Geometry check sheet. Reference: the model listing, model coordinates, mm. A direction names the side the tool comes from. Give positions to 0.01 mm unless a question says otherwise; leave off trailing zeros. Write each loop counter-clockwise with the first axis right and the second up, starting at its lowest first coordinate (ties: lowest second). Pieces come first, ordered by that corner, then holes.
(1) Cross-section at A-A (y = 13). Record the boundary of the cut face in (x, z).
(2) Mould release check, pull along X, two halves, no side actions. Record for faces 1 (the flat face through (-4, 36.037, 2)), 2 (the flat face through (-39.937, 18, 2)), 3 (the flat face through (11, 5.537, 1)), 4 (the flat face through (-3, 31.843, 1)): +X half, -X half, draft (parallel to the pull), parting line (faces both ways), or undercut.
(3) Thickness scan on line 1 along X through (y, z) = (13.5, 0.75); line 2 along Y through (x, z) = (0, 3.35); line 3 along X through (y, z) = (32.5, 0.8). Record the ranges inside material, lowest first.
(4) Cross-section at B-B (x = -14). Record the boundary of the cut face in (y, z).
(5) Depth check by flat-ended pin: P1, Ø3.5, axis at x = -17.22, y = 30.78, coming from the -Z side; P2, Ø12, axis at x = -14.5, y = 17.5, coming from the +Z side; P3, Ø0.8, axis at x = -26, z = 4, coming from the -Y side; P4, Ø0.5, axis at y = 24.5, z = 4, coming from the -X side. Enter the tip coordinate at first touch or a pass-through.
(6) Cross-section at D-D (x = 25). Record the boundary of the cut face in (y, z), and give its area (3 significant figures).
(7) Cross-section at C-C (z = 2.4). Record the boundary of the cut face in (x, y).
(8) Tool access check on faces 5 (the flat face through (-28, 23, 4.5)), 6 (the flat face through (-19.817, 17, 2)), 7 (the flat face through (-19.582, 17, 1)), 8 (the flat face through (-37, 1.037, 2)). Record the directions out of +Z, -Z, +X, -X, +Y, -Y that give a thin tool (end or side, any length) a straight path to the whole face; none if there is none.
```python
from build123d import *

# Parameters (mm, degrees)
SKETCH3_R           = 1.4
SKETCH3_R_2         = 1
BOSS_EXTRUDE1_DEPTH = 3.5
SKETCH9_W           = 33.2
SKETCH9_H           = 33.2
CUT_EXTRUDE1_DEPTH  = 2.2
SKETCH10_W          = 20
SKETCH10_H          = 2.5
CUT_EXTRUDE2_DEPTH  = 1.75
SKETCH11_R          = 1
BOSS_EXTRUDE2_DEPTH = 1
SKETCH14_R          = 3.1
CUT_EXTRUDE3_DEPTH  = 1
SKETCH15_W          = 6.5
SKETCH15_H          = 2
CUT_EXTRUDE4_DEPTH  = 54.906325173


with BuildPart() as part:
    # Sketch3 → Boss-Extrude1 (new body)
    with BuildSketch(Plane.XY):
        Polygon((-39.936821352, -0.962627815), (-39.936821352, 36.037372185), (33.503178648, 36.037372185), (33.503178648, -0.962627815), (7.298178648, -0.962627815), (-14.831821352, -0.962627815), align=None)
        with Locations((-17.216821352, 30.777902568)):
            Circle(SKETCH3_R, mode=Mode.SUBTRACT)
        with Locations((-36.936821352, 32.642902568)):
            Circle(SKETCH3_R_2, mode=Mode.SUBTRACT)
        with Locations((-23.426821352, 32.642902568)):
            Circle(SKETCH3_R_2, mode=Mode.SUBTRACT)
        with Locations((16.993178648, 32.642902568)):
            Circle(SKETCH3_R_2, mode=Mode.SUBTRACT)
        with Locations((30.503178648, 32.642902568)):
            Circle(SKETCH3_R_2, mode=Mode.SUBTRACT)
        with Locations((-17.216821352, 2.777902568)):
            Circle(SKETCH3_R, mode=Mode.SUBTRACT)
        with Locations((10.783178648, 30.777902568)):
            Circle(SKETCH3_R, mode=Mode.SUBTRACT)
        with Locations((10.783178648, 2.777902568)):
            Circle(SKETCH3_R, mode=Mode.SUBTRACT)
        Polygon((-14.981821352, 0.537372185), (-14.981821352, 5.537372185), (-19.581821352, 5.537372185), (-19.581821352, 27.842902568), (-14.981821352, 27.842902568), (-14.981821352, 29.342902568), (8.548178648, 29.342902568), (8.548178648, 27.842902568), (13.148178648, 27.842902568), (13.148178648, 5.537372185), (8.548178648, 5.537372185), (8.548178648, 0.537372185), align=None, mode=Mode.SUBTRACT)
    extrude(amount=BOSS_EXTRUDE1_DEPTH)

    # Sketch9 → Cut-Extrude1 (cut)
    with BuildSketch(Plane(origin=(0, 0, 3.5), x_dir=(-1, 0, 0), z_dir=(0, 0, -1))):
        with Locations((3.216821352, 16.777902568)):
            Rectangle(SKETCH9_W, SKETCH9_H)
    extrude(amount=CUT_EXTRUDE1_DEPTH, mode=Mode.SUBTRACT)

    # Sketch10 → Cut-Extrude2 (cut)
    with BuildSketch(Plane(origin=(0, 0, 0), x_dir=(-1, 0, 0), z_dir=(0, 0, -1))):
        with Locations((3.216821352, 30.592902568)):
            Rectangle(SKETCH10_W, SKETCH10_H)
    extrude(amount=-CUT_EXTRUDE2_DEPTH, mode=Mode.SUBTRACT)

    # Sketch11 → Boss-Extrude2 (add)
    with BuildSketch(Plane.XY.offset(3.5)):
        with BuildLine():
            Line((-34.636821352, 30.942902568), (-34.636821352, 10.942902568))
            Line((-34.636821352, 10.942902568), (-22.636821352, 10.942902568))
            Line((-22.636821352, 10.942902568), (-22.636821352, 30.942902568))
            Line((-22.636821352, 30.942902568), (-21.751928528, 30.942902568))
            ThreePointArc((-21.751928528, 30.942902568), (-21.800520269, 31.226847518), (-21.826821352, 31.513717078))
            Line((-21.826821352, 31.513717078), (-21.826821352, 34.342902568))
            Line((-21.826821352, 34.342902568), (-34.636821352, 34.342902568))
            Line((-34.636821352, 34.342902568), (-34.636821352, 30.942902568))
        make_face()
        with Locations((-23.426821352, 32.642902568)):
            Circle(SKETCH11_R, mode=Mode.SUBTRACT)
    boss_extrude2 = extrude(amount=BOSS_EXTRUDE2_DEPTH)

    # Mirror1: Boss-Extrude2 across plane
    add(boss_extrude2.mirror(Plane.ZY.offset(3.216821352)))

    # Sketch14 → Cut-Extrude3 (cut)
    with BuildSketch(Plane.XY.offset(4.5)):
        with Locations((17.142214959, 27.392343087)):
            Circle(SKETCH14_R)
    extrude(amount=-CUT_EXTRUDE3_DEPTH, mode=Mode.SUBTRACT)

    # Sketch15 → Cut-Extrude4 (cut, through all)
    with BuildSketch(Plane.XY.offset(3.5)):
        with Locations((-36.686821352, 0.037372185)):
            Rectangle(SKETCH15_W, SKETCH15_H)
        with Locations((30.253178648, 0.037372185)):
            Rectangle(SKETCH15_W, SKETCH15_H)
    extrude(amount=-CUT_EXTRUDE4_DEPTH, mode=Mode.SUBTRACT)


solid = part.part
```
Reply:
1. outline: (-39.94, 0) - (-19.58, 0) - (-19.58, 1.3) - (-19.82, 1.3) - (-19.82, 3.5) - (-22.64, 3.5) - (-22.64, 4.5) - (-34.64, 4.5) - (-34.64, 3.5) - (-39.94, 3.5) - close; (13.15, 0) - (33.5, 0) - (33.5, 3.5) - (28.2, 3.5) - (28.2, 4.5) - (16.2, 4.5) - (16.2, 3.5) - (13.38, 3.5) - (13.38, 1.3) - (13.15, 1.3) - close
2. face 1: draft
2. face 2: -X half
2. face 3: undercut
2. face 4: undercut
3. line 1: x = -39.94 to -19.58, 13.15 to 33.5
3. line 2: y = -0.96 to 0.18, 33.38 to 36.04
3. line 3: x = -39.94 to -37.93, -35.95 to -24.42, -22.44 to 16, 17.98 to 29.51, 31.49 to 33.5
4. outline: (-0.96, 0) - (0.54, 0) - (0.54, 1.3) - (0.18, 1.3) - (0.18, 3.5) - (-0.96, 3.5) - close; (29.34, 0) - (36.04, 0) - (36.04, 3.5) - (33.38, 3.5) - (33.38, 1.3) - (29.34, 1.3) - close
5. P1: stops at z = 0
5. P2: stops at z = 3.5
5. P3: stops at y = 10.94
5. P4: stops at x = -34.64
6. outline: (-0.96, 0) - (36.04, 0) - (36.04, 3.5) - (34.34, 3.5) - (34.34, 4.5) - (10.94, 4.5) - (10.94, 3.5) - (-0.96, 3.5) - close
6. area: 153 mm2
7. outline: (-39.94, 1.04) - (-33.44, 1.04) - (-33.44, -0.96) - (27, -0.96) - (27, 1.04) - (33.5, 1.04) - (33.5, 36.04) - (-39.94, 36.04) - close; hole circle Ø2 at (-36.94, 32.64); hole circle Ø2 at (-23.43, 32.64); hole (-19.82, 0.18) - (13.38, 0.18) - (13.38, 33.38) - (-19.82, 33.38) - close; hole circle Ø2 at (16.99, 32.64); hole circle Ø2 at (30.5, 32.64)
8. face 5: +Z, +X, -X, +Y, -Y
8. face 6: +Z
8. face 7: +Z, -Z
8. face 8: +Z, -Z, -X, -Y
